Work out the finished part from the listing and answer in its coordinate system (mm). A direction names the side the tool comes from. Coordinates: 2 decimals unless noted, no trailing zeros. Order: outer loops, then holes, each group sorted by start corner. A loop starts at its lowest first (then second) coordinate and runs counter-clockwise, first axis right, second up. Notation, with made-up numbers: M 11,81.5 L 63,81.5 A22 cw 63,89.5 Z; hole C 58,-7.5 d2. An arc over 180 degrees is marked long. Answer in a Markdown table with one row per item. Add a question column.
Item 1: The part is cut by section C-C (z = -15). Write down the section's boundary in (x, y), then the cut area to 3 significant figures.
Item 2: Consider line 1 (Z direction, x = 298.5, y = 95.9); line 2 (Z direction, x = 300.75, y = 38); line 3 (Y direction, x = 301.5, z = -16). Determine where each line is inside the solid, lowest interval first. Write a range as from..to.
Item 3: The part is cut by section B-B (x = 303.5). Write down the section's boundary in (y, z), then the cut area to 3 significant figures.
Item 4: The part is cut by section A-A (y = 20). Write down the section's boundary in (x, z).
Item 5: The part is cut by section D-D (x = 298.5). Write down the section's boundary in (y, z), then the cut area to 3 significant figures.
Item 6: Flat-ended cylindrical pins translate along their axes: pin 1 Ø6.5 at (x, z) = (298.5, -25) entering from +Y; pin 2 Ø4.5 at (x, z) = (298.5, -25) entering from -Y; pin 3 Ø2.5 at (y, z) = (20, -32) entering from -X. Find the tip coordinate at first contact, or state that the pin passes through.
Item 7: Which of the six approach directions +Z, -Z, +X, -X, +Y, -Y give full straight-line access (tool end or side, diameter ignored) to faces 5 (the face through (298, 7, -25)), 6 (the face through (311.01, 81.88, -29.05)), 7 (the face through (299, 98, -15)), 8 (the face through (299, 2, -15))?
Item 8: The mould has two halves that part along X. Classify faces 1 (the face through (298, 7, -5)), 2 (the face through (300.1, 95.5, -6.2)), 3 (the face through (305, 51, -35)), 4 (the face through (310, 21, -33)): released by +X, released by -X, zero draft, split by the parting line, or undercut.
from build123d import *

# Parameters (mm, degrees)
SKETCH005_W             = 10
SKETCH005_H             = 100
PAD003_DEPTH            = 45
SKETCH006_W             = 10
SKETCH006_H             = 100
POCKET002_DEPTH         = 5
SKETCH007_W             = 96
SKETCH007_H             = 29
PAD004_DEPTH            = 7
SKETCH014_R             = 1
POCKET007_DEPTH         = 10
SKETCH015_R             = 3.5
POCKET008_DEPTH         = 2
SKETCH016_R             = 2
POCKET009_DEPTH         = 5
SKETCH017_R             = 2
POCKET010_DEPTH         = 5
FILLET001_R             = 1
BODY003_PLACEMENT_ANGLE = 180


with BuildPart() as part:
    # Sketch005 → Pad003 (new body)
    with BuildSketch(Plane.XY):
        with Locations((5, 50)):
            Rectangle(SKETCH005_W, SKETCH005_H)
    extrude(amount=PAD003_DEPTH)

    # Sketch006 (on Face5 of Pad003) → Pocket002 (cut)
    with BuildSketch(Plane(origin=(0, 0, 0), x_dir=(1, 0, 0), z_dir=(0, 0, -1))):
        with Locations((10, -50)):
            Rectangle(SKETCH006_W, SKETCH006_H)
    extrude(amount=-POCKET002_DEPTH, mode=Mode.SUBTRACT)

    # Sketch007 (on Face5 of Pocket002) → Pad004 (join)
    with BuildSketch(Plane.YZ.offset(10)):
        with Locations((50, 25.5)):
            Rectangle(SKETCH007_W, SKETCH007_H)
    extrude(amount=PAD004_DEPTH)

    # Sketch014 (on Face7 of Pad004) → Pocket007 (cut)
    with BuildSketch(Plane(origin=(0, 0, 0), x_dir=(0, -1, 0), z_dir=(-1, 0, 0))):
        with Locations((-20, 8)):
            Circle(SKETCH014_R)
        with Locations((-80, 8)):
            Circle(SKETCH014_R)
    extrude(amount=-POCKET007_DEPTH, mode=Mode.SUBTRACT)

    # Sketch015 (on Face7 of Pocket007) → Pocket008 (cut)
    with BuildSketch(Plane(origin=(0, 0, 0), x_dir=(0, -1, 0), z_dir=(-1, 0, 0))):
        with Locations((-20, 8)):
            Circle(SKETCH015_R)
        with Locations((-80, 8)):
            Circle(SKETCH015_R)
    extrude(amount=-POCKET008_DEPTH, mode=Mode.SUBTRACT)

    # Sketch016 (on Face9 of Pocket008) → Pocket009 (cut)
    with BuildSketch(Plane.XZ.offset(-2)):
        with Locations((13.5, 15)):
            Circle(SKETCH016_R)
        with Locations((13.5, 35)):
            Circle(SKETCH016_R)
    extrude(amount=-POCKET009_DEPTH, mode=Mode.SUBTRACT)

    # Sketch017 (on Face12 of Pocket009) → Pocket010 (cut)
    with BuildSketch(Plane(origin=(0, 98, 0), x_dir=(-1, 0, 0), z_dir=(0, 1, 0))):
        with Locations((-13.5, 15)):
            Circle(SKETCH017_R)
        with Locations((-13.5, 35)):
            Circle(SKETCH017_R)
    extrude(amount=-POCKET010_DEPTH, mode=Mode.SUBTRACT)

    # Fillet001
    fillet001_edges = [part.edges().sort_by_distance(p)[0] for p in [
        (5, 0, 45),
        (5, 100, 45),
    ]]
    fillet(fillet001_edges, radius=FILLET001_R)


with BuildPart() as part_1:
    # Body002 placement: moved
    add(part.part.moved(Location((-10, 0, -40))))


with BuildPart() as part_2:
    # Body003 placement: moved
    add(part_1.part.moved(Location((302, 100, 0))).rotate(Axis((302, 100, 0), (0, 0, 1)), BODY003_PLACEMENT_ANGLE))


solid = part_2.part
Reply:
| question | item | result |
|---|---|---|
| 1 | outline | M 295,2 L 302,2 L 302,0 L 312,0 L 312,100 L 302,100 L 302,98 L 295,98 Z |
| 1 | area | 1,670 mm2 |
| 2 | line 1 | z = -29..-27, -23..-7, -3..0 |
| 2 | line 2 | z = -29..0 |
| 2 | line 3 | y = 2..98 |
| 3 | outline | M 0,-35 L 100,-35 L 100,4 A1 ccw 99,5 L 1,5 A1 ccw 0,4 Z; hole C 20,-32 d2; hole C 80,-32 d2 |
| 3 | area | 3,990 mm2 |
| 4 | outline | M 295,-29 L 302,-29 L 302,-31 L 310,-31 L 310,-28.5 L 312,-28.5 L 312,5 L 302,5 L 302,0 L 295,0 Z; M 302,-35 L 307,-35 L 307,-40 L 312,-40 L 312,-35.5 L 310,-35.5 L 310,-33 L 302,-33 Z |
| 5 | outline | M 2,-29 L 98,-29 L 98,-27 L 93,-27 L 93,-23 L 98,-23 L 98,-7 L 93,-7 L 93,-3 L 98,-3 L 98,0 L 2,0 L 2,-3 L 7,-3 L 7,-7 L 2,-7 L 2,-23 L 7,-23 L 7,-27 L 2,-27 Z |
| 5 | area | 2,700 mm2 |
| 6 | pin 1 | stops at y = 98 |
| 6 | pin 2 | stops at y = 2 |
| 6 | pin 3 | stops at x = 302 |
| 7 | face 5 | -Y |
| 7 | face 6 | +X |
| 7 | face 7 | +Z, -Z, -X, +Y |
| 7 | face 8 | +Z, -Z, -X, -Y |
| 8 | face 1 | undercut |
| 8 | face 2 | undercut |
| 8 | face 3 | zero draft |
| 8 | face 4 | released by +X |
